Part model, mm, in its own coordinate system. A direction names the side the tool comes from. Coordinates: 2 decimals unless noted, no trailing zeros. Order: outer loops, then holes, each group sorted by start corner. A loop starts at its lowest first (then second) coordinate and runs counter-clockwise, first axis right, second up. Notation, with made-up numbers: (65, -37) - (73, -37) arc R18 cw to (73, -3) - close; hole circle Ø9 at (-21.75, -12.5). An arc over 180 degrees is marked (long way). Use a Markdown table: item, result. Add a question column.
1) Two-plate mould, pull along X, no slides. Class faces 1 (the face through (-78, 32, 2)), 2 (the face through (40, 44, 2)), 3 (the face through (76, 24, 2)), 4 (the face through (-45, 42, 2)): +X half, -X half, draft (parallel to the pull), parting line (faces both ways), or undercut.
2) Drop flat-ended pins along their axis: P1, Ø1, axis at x = 50, z = 3.5, coming from the -Y side; P2, Ø2, axis at y = 27, z = 1, coming from the -X side. Give the stop position or say it passes through.
3) Wall check: L1, parallel to Y at x = 44, z = 1.4; L2, parallel to X at y = 8, z = 2.4; L3, parallel to X at y = 30, z = 1.9. Give the ranges that are in metal, low to high. Write a range as [from, to].
4) Saw through at A-A on y = 38. List the corners of the cut face in (x, z).
5) Saw through at D-D on x = -8.5. List the corners of the cut face in (y, z).
6) Saw through at C-C on z = 3.25. Count the separate pieces of the cut face and the enclosed holes in it, then the cut area to 3 significant figures.
7) Tool access for faces 5 (the face through (-70, 46, 2)), 6 (the face through (57, 42, 2)), 7 (the face through (15, -2, 2)), 8 (the face through (27, -4, 2)), 9 (the face through (78, 16, 2)): list every direction of +Z, -Z, +X, -X, +Y, -Y with a clear straight run to the whole face (end or side of a thin tool).
8) Saw through at B-B on x = 44. List the corners of the cut face in (y, z), then the cut area to 3 significant figures.
Autodesk Inventor part; units mm, degrees
ref_plane "YZ Plane" through (0, 0, 0) normal (1, 0, 0) x (0, 1, 0)
ref_plane "XZ Plane" through (0, 0, 0) normal (0, 1, 0) x (-1, 0, 0)
ref_plane "XY Plane" through (0, 0, 0) normal (0, 0, 1) x (1, 0, 0)
sketch "Эскиз1" plane through (0, 0, 0) normal (0, 0, 1) x (1, 0, 0)
  line L0 (0, 0) -> (-15, 0)
  line L1 (-15, 0) -> (-15, -4)
  line L2 (-15, -4) -> (-40, -4)
  line L3 (-40, -4) -> (-40, 0)
  line L4 (-40, 0) -> (-49, 0)
  line L5 (-49, 0) -> (-49, 9)
  line L6 (-49, 9) -> (-53, 9)
  line L7 (-53, 9) -> (-53, -4)
  line L8 (-53, -4) -> (-80, -4)
  line L9 (-80, 46) -> (-60, 46)
  line L10 (-60, 46) -> (-60, 42)
  line L11 (-60, 42) -> (-53, 42)
  line L12 (-53, 42) -> (-53, 29)
  line L13 (-53, 29) -> (-49, 29)
  line L14 (-49, 29) -> (-49, 42)
  line L15 (-49, 42) -> (-40, 42)
  line L16 (-40, 42) -> (-40, 46)
  line L17 (-40, 46) -> (-15, 46)
  line L18 (-15, 46) -> (-15, 42)
  line L19 (-15, 42) -> (0, 42)
  line L20 (0, 42) -> (0, 0)
  line L21 (0, 0) -> (15, 0)
  line L22 (15, 0) -> (15, -4)
  line L23 (15, -4) -> (40, -4)
  line L24 (40, -4) -> (40, 0)
  line L25 (40, 0) -> (49, 0)
  line L26 (49, 0) -> (49, 9)
  line L27 (49, 9) -> (53, 9)
  line L28 (53, 9) -> (53, -4)
  line L29 (53, -4) -> (80, -4)
  line L30 (80, 46) -> (60, 46)
  line L31 (60, 46) -> (60, 42)
  line L32 (60, 42) -> (53, 42)
  line L33 (53, 42) -> (53, 29)
  line L34 (53, 29) -> (49, 29)
  line L35 (49, 29) -> (49, 42)
  line L36 (49, 42) -> (40, 42)
  line L37 (40, 42) -> (40, 46)
  line L38 (40, 46) -> (15, 46)
  line L39 (15, 46) -> (15, 42)
  line L40 (15, 42) -> (0, 42)
  line L41 (-80, -4) -> (-80, 16)
  line L42 (-80, 16) -> (-76, 16)
  line L43 (-76, 16) -> (-76, 32)
  line L44 (-76, 32) -> (-80, 32)
  line L45 (-80, 32) -> (-80, 46)
  line L46 (80, -4) -> (80, 16)
  line L47 (76, 16) -> (76, 32)
  line L48 (76, 32) -> (80, 32)
  line L49 (80, 16) -> (76, 16)
  line L50 (80, 32) -> (80, 46)
  dimension "d0" = 4
  dimension "d1" = 30
  dimension "d2" = 25
  dimension "d3" = 9
  dimension "d4" = 20
  dimension "d5" = 13
  dimension "d6" = 17
  dimension "d9" = 25
  dimension "d12" = 20
  dimension "d13" = 27
  dimension "d14" = 16
  dimension "d15" = 14
extrude "Выдавливание1" add sketch "Эскиз1" along normal blind 4
sketch "Эскиз3" plane through (0, 0, 4) normal (0, 0, 1) x (1, 0, 0)
  line L0 (0, 0) -> (0, 42)
  line L1 (15, 42) -> (-15, 42)
  line L2 (-40, 42) -> (-49, 42)
  line L3 (-49, 42) -> (-49, 29)
  point P0 (-44, 30)
  point P1 (-44, 8)
  point P2 (44, 8)
  point P3 (44, 30)
  dimension "d28" = 12
  dimension "d29" = 34
  dimension "d30" = 5
hole "Отверстие1" at (-44, 30, 4) at (-44, 8, 4) at (44, 8, 4) at (44, 30, 4) direction (0, 0, -1) diameter 2.8 end through all
properties part number "back" material "Дерево (береза)"
Results are:
| question | item | result |
|---|---|---|
| 1 | face 1 | draft |
| 1 | face 2 | undercut |
| 1 | face 3 | +X half |
| 1 | face 4 | undercut |
| 2 | P1 | y = 9 |
| 2 | P2 | x = -76 |
| 3 | L1 | [0, 6.6], [9.4, 28.6], [31.4, 42] |
| 3 | L2 | [-80, -53], [-49, -45.4], [-42.6, 42.6], [45.4, 49], [53, 80] |
| 3 | L3 | [-76, -53], [-49, -45.4], [-42.6, 42.6], [45.4, 49], [53, 76] |
| 4 | outline | (-80, 0) - (-53, 0) - (-53, 4) - (-80, 4) - close; (-49, 0) - (49, 0) - (49, 4) - (-49, 4) - close; (53, 0) - (80, 0) - (80, 4) - (53, 4) - close |
| 5 | outline | (0, 0) - (42, 0) - (42, 4) - (0, 4) - close |
| 6 | separate pieces | 1 |
| 6 | enclosed holes | 4 |
| 6 | area | 7,170 mm2 |
| 7 | face 5 | +Z, -Z, +X, -X, +Y |
| 7 | face 6 | +Z, -Z, +Y |
| 7 | face 7 | +Z, -Z, -Y |
| 7 | face 8 | +Z, -Z, +X, -X, -Y |
| 7 | face 9 | +Z, -Z, +X |
| 8 | outline | (0, 0) - (6.6, 0) - (6.6, 4) - (0, 4) - close; (9.4, 0) - (28.6, 0) - (28.6, 4) - (9.4, 4) - close; (31.4, 0) - (42, 0) - (42, 4) - (31.4, 4) - close |
| 8 | area | 146 mm2 |
